Source: CAD feature listing. Evaluate the final solid. Frame: model axes, mm. A direction names the side the tool comes from. Round coordinates to 2 decimals unless told otherwise and drop trailing zeros. Loops run counter-clockwise (first coordinate to the right, second up) from the corner with the lowest first, then second, coordinate; pieces in that order, holes last. Notation, with made-up numbers: M 73,65.5 L 96,65.5 A16 ccw 96,85.5 Z; hole C 4,37 d4. An arc over 180 degrees is marked long. Write each question's results on one line, items separated by ' | '. Start each with the question number.
1. Ray query, line 1 (X direction, y = 61, z = 0); line 2 (X direction, y = 104, z = 133). Return the intervals inside material, ascending.
2. Section C-C on x = -178. Output: boundary loops of the cut face in (y, z), and give its area (3 significant figures).
3. Contact query for flat-ended pins moving along their axis: pin 1 Ø6 at (x, y) = (-103.5, 30.5) entering from -Z; pin 2 Ø4 at (y, z) = (162, 144.5) entering from +X. Output: stop coordinate, or through.
4. Section A-A on y = 94.5. Output: boundary loops of the cut face in (x, z).
5. Set-up query: faces 1 (the conical face through (72.381, 264.303, 30.011)), 2 (the flat face through (164.51, 190.98, -0.02)), 3 (the flat face through (1.5, 99, 148)), 4 (the flat face through (1.5, 99, -164)), 5 (the flat face through (-148, 99, 1.5)). Return all of +Z, -Z, +X, -X, +Y, -Y with unobstructed straight access to the full face (end or side cutting, diameter ignored); none if empty.
6. Draft query along X for faces 6 (the flat face through (-1.5, 99, 164)), 7 (the flat face through (-164, 99, -1.5)), 8 (the cylindrical face through (23.49, 130.47, 74.59)). Return one class per face: released by +X, released by -X, zero draft, split by the parting line, or undercut.
7. Section D-D on z = -195. Output: boundary loops of the cut face in (x, y), and give its area (3 significant figures).
8. Section B-B on y = 214.5. Output: boundary loops of the cut face in (x, z), and give its area (3 significant figures).
from build123d import *

# Parameters (mm, degrees)
SKETCH1_R                = 80.7
SKETCH1_R_2              = 78.2
BOSS_EXTRUDE1_DEPTH      = 260
BOSS_EXTRUDE2_DEPTH      = 1.5
BOSS_EXTRUDE2_DEPTH_BACK = 1.5
BOSS_EXTRUDE3_DEPTH      = 1.5
BOSS_EXTRUDE3_DEPTH_BACK = 1.5
SKETCH4_W                = 2
SKETCH4_H                = 260
CIRPATTERN1_COUNT        = 4
SKETCH6_R                = 78.2
BOSS_EXTRUDE4_DEPTH      = 10
CHAMFER1_START           = 264.638732699
CHAMFER1_2_OUTLINE_R     = 80.7
CHAMFER1_2_OUTLINE_R_2   = 78.2
CHAMFER1_2_DEPTH         = 5.361267301
CHAMFER1_START_2         = 258
CHAMFER1_3_DEPTH         = 2


with BuildPart() as part:
    # Sketch1 → Boss-Extrude1 (new body)
    with BuildSketch(Plane(origin=(0, 0, 0), x_dir=(1, 0, 0), z_dir=(0, 1, 0))):
        with Locations(Location((0, 0, 0), (0, 0, 270))):
            Circle(SKETCH1_R)
        with Locations(Location((0, 0, 0), (0, 0, 270))):
            Circle(SKETCH1_R_2, mode=Mode.SUBTRACT)
    extrude(amount=BOSS_EXTRUDE1_DEPTH)



with BuildPart() as body_2:
    # Sketch2 → Boss-Extrude2 (new, two sides: drawn at the far end of the back side and taken through both)
    with BuildSketch(Plane.XY.offset(-BOSS_EXTRUDE2_DEPTH_BACK)):
        Polygon((80.7, 0), (80.7, 260), (250.7, 120), (250.7, 0), align=None)
    extrude(amount=BOSS_EXTRUDE2_DEPTH + BOSS_EXTRUDE2_DEPTH_BACK)


with BuildPart() as part_1:
    add(part.part)

    add(body_2.part)  # Boss-Extrude3 merges body 2
    # Sketch4 → Boss-Extrude3 (add, two sides: drawn at the far end of the back side and taken through both)
    with BuildSketch(Plane.XY.offset(-BOSS_EXTRUDE3_DEPTH_BACK)):
        with Locations((79.7, 130)):
            Rectangle(SKETCH4_W, SKETCH4_H)
    extrude(amount=BOSS_EXTRUDE3_DEPTH + BOSS_EXTRUDE3_DEPTH_BACK)


with BuildPart() as cirpattern1_1:
    # CirPattern1: pattern copy
    add(part_1.part.rotate(Axis((0, 0, 0), (0, 1, 0)), 1 * 360 / CIRPATTERN1_COUNT))


with BuildPart() as cirpattern1_2:
    # CirPattern1: pattern copy
    add(part_1.part.rotate(Axis((0, 0, 0), (0, 1, 0)), 2 * 360 / CIRPATTERN1_COUNT))


with BuildPart() as cirpattern1_3:
    # CirPattern1: pattern copy
    add(part_1.part.rotate(Axis((0, 0, 0), (0, 1, 0)), 3 * 360 / CIRPATTERN1_COUNT))


with BuildPart() as part_2:
    add(part_1.part)

    add(cirpattern1_1.part)  # Boss-Extrude4 merges CirPattern1_1

    add(cirpattern1_2.part)  # Boss-Extrude4 merges CirPattern1_2

    add(cirpattern1_3.part)  # Boss-Extrude4 merges CirPattern1_3
    # Sketch6 → Boss-Extrude4 (add)
    with BuildSketch(Plane(origin=(0, 260, 0), x_dir=(1, 0, 0), z_dir=(0, 1, 0))):
        with BuildLine():
            ThreePointArc((80.686058275, -1.5), (80.7, 0), (80.686058275, 1.5))
            ThreePointArc((80.686058275, 1.5), (57.063517242, 57.063517242), (1.5, 80.686058275))
            ThreePointArc((1.5, 80.686058275), (0, 80.7), (-1.5, 80.686058275))
            ThreePointArc((-1.5, 80.686058275), (-57.063517242, -57.063517242), (80.686058275, -1.5))
        make_face()
        with Locations(Location((0, 0, 0), (0, 0, 270))):
            Circle(SKETCH6_R, mode=Mode.SUBTRACT)
    extrude(amount=BOSS_EXTRUDE4_DEPTH)

    # Chamfer1: read off the stored shape, not the designer's step
    # Chamfer1 outline → Chamfer1 (revolve, cut)
    with BuildSketch(Plane.XY):
        Polygon((78.2, 264.638732699), (80.7, 259.277465397), (80.7, 264.638732699), align=None)
    revolve(axis=Axis((0, 0, 0), (0, 1, 0)), mode=Mode.SUBTRACT)

    # Chamfer1 2 outline → Chamfer1 2 (cut)
    with BuildSketch(Plane(origin=(0, 0, 0), x_dir=(1, 0, 0), z_dir=(0, 1, 0)).offset(CHAMFER1_START)):
        Circle(CHAMFER1_2_OUTLINE_R)
        Circle(CHAMFER1_2_OUTLINE_R_2, mode=Mode.SUBTRACT)
    extrude(amount=CHAMFER1_2_DEPTH, mode=Mode.SUBTRACT)

    # Chamfer1 3 outline → Chamfer1 3 (add)
    with BuildSketch(Plane(origin=(0, 0, 0), x_dir=(1, 0, 0), z_dir=(0, 1, 0)).offset(CHAMFER1_START_2)):
        with BuildLine():
            ThreePointArc((80.686058275, -1.5), (80.7, 0), (80.686058275, 1.5))
            Line((80.686058275, 1.5), (80.349076396, 1.5))
            ThreePointArc((80.349076396, 1.5), (80.363076582, 0), (80.349076396, -1.5))
            Line((80.349076396, -1.5), (80.686058275, -1.5))
        make_face()
        with BuildLine():
            Line((1.5, 80.349076396), (1.5, 80.686058275))
            ThreePointArc((1.5, 80.686058275), (0, 80.7), (-1.5, 80.686058275))
            Line((-1.5, 80.686058275), (-1.5, 80.349076396))
            ThreePointArc((-1.5, 80.349076396), (0, 80.363076582), (1.5, 80.349076396))
        make_face()
        with BuildLine():
            ThreePointArc((-1.5, -80.686058275), (0, -80.7), (1.5, -80.686058275))
            Line((1.5, -80.686058275), (1.5, -80.349076396))
            ThreePointArc((1.5, -80.349076396), (0, -80.363076582), (-1.5, -80.349076396))
            Line((-1.5, -80.349076396), (-1.5, -80.686058275))
        make_face()
        with BuildLine():
            Line((-80.349076396, 1.5), (-80.686058275, 1.5))
            ThreePointArc((-80.686058275, 1.5), (-80.7, 0), (-80.686058275, -1.5))
            Line((-80.686058275, -1.5), (-80.349076396, -1.5))
            ThreePointArc((-80.349076396, -1.5), (-80.363076582, 0), (-80.349076396, 1.5))
        make_face()
    extrude(amount=CHAMFER1_3_DEPTH)


solid = part_2.part
Taken from the geometry:
1) line 1: -250.7 to -78.2, 78.2 to 250.7 | line 2: -1.5 to 1.5
2) outline: M 0,-1.5 L 179.87,-1.5 L 179.87,1.5 L 0,1.5 Z | area: 540 mm^2
3) pin 1: z = -1.5 | pin 2: x = 1.5
4) outline: M -250.7,-1.5 L -80.69,-1.5 A80.7 ccw -1.5,-80.69 L -1.5,-250.7 L 1.5,-250.7 L 1.5,-80.69 A80.7 ccw 80.69,-1.5 L 250.7,-1.5 L 250.7,1.5 L 80.69,1.5 A80.7 ccw 1.5,80.69 L 1.5,250.7 L -1.5,250.7 L -1.5,80.69 A80.7 ccw -80.69,1.5 L -250.7,1.5 Z; hole C 0,0 d156.4
5) face 1: +Y | face 2: +Z, -Z, +X, +Y | face 3: +Z, +X, +Y, -Y | face 4: -Z, +X, +Y, -Y | face 5: +Z, -X, +Y, -Y
6) face 6: released by -X | face 7: zero draft | face 8: undercut
7) outline: M -1.5,0 L 1.5,0 L 1.5,165.87 L -1.5,165.87 Z | area: 498 mm^2
8) outline: M -135.95,-1.5 L -80.69,-1.5 A80.7 ccw -1.5,-80.69 L -1.5,-135.95 L 1.5,-135.95 L 1.5,-80.69 A80.7 ccw 80.69,-1.5 L 135.95,-1.5 L 135.95,1.5 L 80.69,1.5 A80.7 ccw 1.5,80.69 L 1.5,135.95 L -1.5,135.95 L -1.5,80.69 A80.7 ccw -80.69,1.5 L -135.95,1.5 Z; hole C 0,0 d156.4 | area: 1,910 mm^2
